Build history of the part. All positions in model axes, mm. A direction names the side the tool comes from. Round coordinates to 2 decimals unless told otherwise and drop trailing zeros. Write each loop counter-clockwise with the first axis right and the second up, starting at its lowest first coordinate (ties: lowest second). Pieces come first, ordered by that corner, then holes. Notation, with made-up numbers: M 47.5,6.5 L 64.5,6.5 A19 ccw 64.5,31.5 Z; hole C -7,62.5 d9. An arc over 180 degrees is marked long. Write item = value, one per line. Start each with the question number.
Q1. Band-saw the part on B-B on x = 20. Write the cut outline in (y, z).
Q2. Tool access for faces 5 (the flat face through (2, -25.4, -9)), 6 (the flat face through (-8.281, -13, 27)), 7 (the flat face through (17.383, -23, -42)), 8 (the flat face through (-15, -13, 38.951)), 9 (the flat face through (22, -13, -35.392)): list every direction of +Z, -Z, +X, -X, +Y, -Y with a clear straight run to the whole face (end or side of a thin tool).
Q3. Band-saw the part on D-D on z = -24. Write the cut outline in (x, y).
Q4. Drop flat-ended pins along their axis: P1, Ø5, axis at x = 10, y = -24, coming from the +Z side; P2, Ø1, axis at y = -18.5, z = -35.5, coming from the +X side; P3, Ø3.5, axis at y = -19.5, z = -42.5, coming from the +X side. Give the stop position or say it passes through.
Q5. Band-saw the part on C-C on y = -7. Write the cut outline in (x, z), plus the area to 3 significant figures.
Q6. Pull direction X, two halves, no side cores. Call faces 1 (the flat face through (14.749, -13, 27)), 2 (the cylindrical face through (2.981, -12.878, 2.906)), 3 (the flat face through (22, -46.427, -43)), 4 (the flat face through (26.395, -13, 1)): released by +X, released by -X, zero draft, split by the parting line, or undercut.
Q7. Probe L1, parallel to X at y = -14.5, z = -31; L2, parallel to Z at x = 3, y = -63.5; L3, parallel to X at y = -16, z = 24. List the from-to ranges inside material, lowest first.
Q8. Band-saw the part on A-A on z = 16.5. Write the cut outline in (x, y).
```python
from build123d import *

# Parameters (mm, degrees)
F0_W     = 48.2076276094
F0_H     = 85.6006219983
F1_DEPTH = 25.4
F3_DEPTH = 25.4
F4_W     = 10.3362295777
F4_H     = 11.2576633692
F4_W_2   = 2.2321604192
F5_DEPTH = 25.4
F7_DEPTH = 6.858


with BuildPart() as f1:
    # F0 (on Front) → F1 (new body)
    with BuildSketch(Plane.XZ):
        with Locations((2.2912370041, -3.8492791355)):
            Rectangle(F0_W, F0_H)
    extrude(amount=F1_DEPTH)

    # F2 (on face) → F3 (cut)
    with BuildSketch(Plane.XZ.offset(25.4)):
        with BuildLine():
            Line((14.7487549111, 38.9510318637), (-8.2807904109, 38.9510318637))
            Line((-8.2807904109, 38.9510318637), (-8.2807904109, 14.4174993038))
            ThreePointArc((-8.2807904109, 14.4174993038), (3.2339822501, 2.9027266428), (14.7487549111, 14.4174993038))
            Line((14.7487549111, 14.4174993038), (14.7487549111, 38.9510318637))
        make_face()
    extrude(amount=-F3_DEPTH, mode=Mode.SUBTRACT)

    # F4 (on face) → F5 (cut)
    with BuildSketch(Plane.XZ.offset(25.4)):
        with Locations((22.5512860343, -41.02075845)):
            Rectangle(F4_W, F4_H)
        with Locations((28.8354810327, -41.02075845)):
            Rectangle(F4_W_2, F4_H)
    extrude(amount=-F5_DEPTH, mode=Mode.SUBTRACT)

    # F6 (on face) → F7 (join)
    with BuildSketch(Plane(origin=(0, 0, -46.6495901346), x_dir=(1, 0, 0), z_dir=(0, 0, -1))):
        with BuildLine():
            Line((-21.8125768006, 62.740623951), (-21.8125768006, 25.4))
            Line((-21.8125768006, 25.4), (17.3831712455, 25.4))
            Line((17.3831712455, 25.4), (17.3831712455, 46.4270114899))
            Line((17.3831712455, 46.4270114899), (26.6548879445, 46.4270114899))
            Line((26.6548879445, 46.4270114899), (26.6548879445, 62.740623951))
            ThreePointArc((26.6548879445, 62.740623951), (2.4211555719, 86.9743563235), (-21.8125768006, 62.740623951))
        make_face()
    extrude(amount=-F7_DEPTH)


solid = f1.part
```
Conclusion:
q1.outline = M -79.42,-46.65 L -46.43,-46.65 L -46.43,-39.79 L -79.42,-39.79 Z; M -25.4,-35.39 L 0,-35.39 L 0,38.95 L -25.4,38.95 Z
q2.face_5 = +Z, +X, -X, -Y
q2.face_6 = +Z, +Y, -Y
q2.face_7 = -Z, +X, +Y
q2.face_8 = +Z, +X, -X, +Y, -Y
q2.face_9 = -Z, +X, +Y, -Y
q3.outline = M -21.81,-25.4 L 26.4,-25.4 L 26.4,0 L -21.81,0 Z
q4.P1 = 7.58
q4.P2 = 26.4
q4.P3 = 17.38
q5.outline = M -21.81,-46.65 L 17.38,-46.65 L 17.38,-35.39 L 26.4,-35.39 L 26.4,38.95 L 14.75,38.95 L 14.75,14.42 A11.51 cw -8.28,14.42 L -8.28,38.95 L -21.81,38.95 Z
q5.area = 3,250 mm^2
q6.face_1 = undercut
q6.face_2 = undercut
q6.face_3 = zero draft
q6.face_4 = released by +X
q7.L1 = -21.81 to 26.4
q7.L2 = -46.65 to -39.79
q7.L3 = -21.81 to -8.28, 14.75 to 26.4
q8.outline = M -21.81,-25.4 L -8.28,-25.4 L -8.28,0 L -21.81,0 Z; M 14.75,-25.4 L 26.4,-25.4 L 26.4,0 L 14.75,0 Z
